Verification items for the finished model (mm, model axes). Give positions to 0.01 mm unless a question says otherwise; leave off trailing zeros. Loops run counter-clockwise (first coordinate to the right, second up) from the corner with the lowest first, then second, coordinate; pieces in that order, holes last. Notation, with made-up numbers: M -25.5,77 L -4.5,77 A25 ccw -4.5,106 Z; hole C -38,3 d5. An arc over 180 degrees is marked long. Write each question's results on one line, items separated by ' | '. Start each with the question number.
```python
from build123d import *

# Parameters (mm, degrees)
F0_R     = 17.5
F1_DEPTH = 5
F2_W     = 6.4513552934
F2_H     = 36.834217608
F3_DEPTH = 5
F4_W     = 12.2471041977
F4_H     = 55.2336238325
F5_DEPTH = 25
F7_DEPTH = 25
F8_W     = 30.2105266601
F8_H     = 23.1209599674
F9_DEPTH = 25


with BuildPart() as f1:
    # F0 (on Top) → F1 (new body)
    with BuildSketch(Plane.XY):
        with BuildLine():
            Line((0, 50.2336238325), (0, 0))
            Line((0, 0), (60, 0))
            Line((60, 0), (60, 50.2336238325))
            ThreePointArc((60, 50.2336238325), (58.5355339059, 53.7691577384), (55, 55.2336238325))
            Line((55, 55.2336238325), (5, 55.2336238325))
            ThreePointArc((5, 55.2336238325), (1.4644660941, 53.7691577384), (0, 50.2336238325))
        make_face()
        with Locations((30, 30)):
            Circle(F0_R, mode=Mode.SUBTRACT)
    extrude(amount=F1_DEPTH)

    # F2 (on face) → F3 (join)
    with BuildSketch(Plane.XY.offset(5)):
        with Locations((-3.2256776467, 18.417108804)):
            Rectangle(F2_W, F2_H)
        with BuildLine():
            Line((-6.4513552934, 36.834217608), (0, 36.834217608))
            Line((0, 36.834217608), (0, 50.2336238325))
            ThreePointArc((0, 50.2336238325), (1.4644660941, 53.7691577384), (5, 55.2336238325))
            Line((5, 55.2336238325), (-36.6618819535, 55.2336238325))
            Line((-36.6618819535, 55.2336238325), (-36.6618819535, -38.6209599674))
            Line((-36.6618819535, -38.6209599674), (-6.4513552934, -38.6209599674))
            Line((-6.4513552934, -38.6209599674), (-6.4513552934, 0))
            Line((-6.4513552934, 0), (-6.4513552934, 36.834217608))
        make_face()
    extrude(amount=-F3_DEPTH)

    # F4 (on face) → F5 (cut)
    with BuildSketch(Plane.XY.offset(5)):
        with Locations((60.3161063045, 27.6168119162)):
            Rectangle(F4_W, F4_H)
    extrude(amount=-F5_DEPTH, mode=Mode.SUBTRACT)

    # F6 (on face) → F7 (cut)
    with BuildSketch(Plane.XY.offset(5)):
        with BuildLine():
            ThreePointArc((29.3901374458, 52.9360723045), (46.0069133431, 46.4381893869), (52.9441788934, 30))
            ThreePointArc((52.9441788934, 30), (46.542618257, 14.1010337978), (30.910082361, 7.0738774498))
            Line((30.910082361, 7.0738774498), (30.910082361, 0))
            Line((30.910082361, 0), (54.1925542057, 0))
            Line((54.1925542057, 0), (54.1925542057, 55.2336238325))
            Line((54.1925542057, 55.2336238325), (-36.6618819535, 55.2336238325))
            Line((-36.6618819535, 55.2336238325), (-36.6618819535, 52.9360723045))
            Line((-36.6618819535, 52.9360723045), (29.3901374458, 52.9360723045))
        make_face()
    extrude(amount=-F7_DEPTH, mode=Mode.SUBTRACT)

    # F8 (on face) → F9 (cut)
    with BuildSketch(Plane.XY.offset(5)):
        with Locations((-21.5566186234, -27.0604799837)):
            Rectangle(F8_W, F8_H)
    extrude(amount=-F9_DEPTH, mode=Mode.SUBTRACT)


solid = f1.part
```
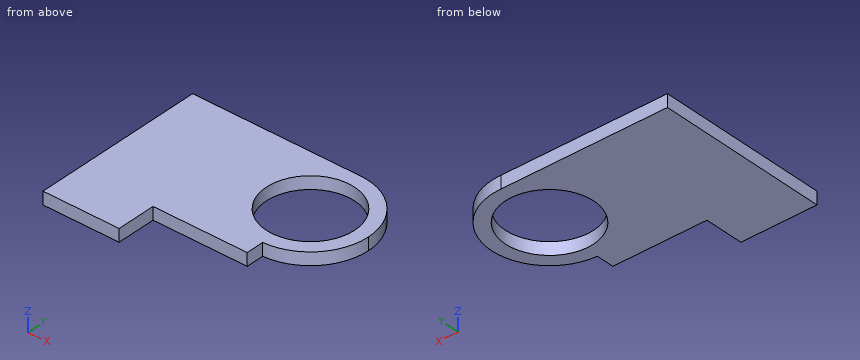
1. Depth check by flat-ended pin: pin 1 Ø2.5 at (x, z) = (10.5, 2) entering from +Y; pin 2 Ø1.5 at (x, z) = (6.5, 3.5) entering from -Y. Enter the tip coordinate at first touch or a pass-through.
2. Section check D-D, the plane y = 5. Record the boundary of the cut face in (x, z).
3. Thickness scan on probe 1 along X at (y, z) = (29.5, 1.9); probe 2 along Y at (x, z) = (30, 2.3); probe 3 along Y at (x, z) = (-1, 4.15). Record the ranges inside material, lowest first.
4. Section check A-A, the plane y = 18.5. Record the boundary of the cut face in (x, z), plus the area to 3 significant figures.
5. Section check B-B, the plane z = 2.5. Record the boundary of the cut face in (x, y), plus the area to 3 significant figures.
6. Section check C-C, the plane x = -4. Record the boundary of the cut face in (y, z).
Filled sheet:
1) pin 1: y = 52.94 | pin 2: y = 0
2) outline: M -36.66,0 L 30.91,0 L 30.91,5 L -36.66,5 Z
3) probe 1: -36.66 to 12.51, 47.49 to 52.94 | probe 2: 0 to 12.5, 47.5 to 52.94 | probe 3: 0 to 52.94
4) outline: M -36.66,0 L 16.81,0 L 16.81,5 L -36.66,5 Z; M 43.19,0 L 49.85,0 L 49.85,5 L 43.19,5 Z | area: 301 mm2
5) outline: M -36.66,-15.5 L -6.45,-15.5 L -6.45,0 L 30.91,0 L 30.91,7.07 A22.94 ccw 29.39,52.94 L -36.66,52.94 Z; hole C 30,30 d35 | area: 3,870 mm2
6) outline: M 0,0 L 52.94,0 L 52.94,5 L 0,5 Z
